from build123d import *

# Parameters (mm, degrees)
SKETCH1_W                      = 80
SKETCH1_H                      = 12.7
BOSS_EXTRUDE1_DEPTH            = 12.7
M4_CLEARANCE_HOLE1_D           = 4.8
M4_CLEARANCE_HOLE1_CSINK_D     = 4.85
M4_CLEARANCE_HOLE1_CSINK_ANGLE = 100
M8_CLEARANCE_HOLE1_D           = 10
M8_CLEARANCE_HOLE1_CSINK_D     = 10.05
M8_CLEARANCE_HOLE1_CSINK_ANGLE = 100
M5_CLEARANCE_HOLE1_D           = 5.8
M5_CLEARANCE_HOLE1_CSINK_D     = 5.85
M5_CLEARANCE_HOLE1_CSINK_ANGLE = 100


with BuildPart() as part:
    # Sketch1 → Boss-Extrude1 (new body)
    with BuildSketch(Plane(origin=(0, 0, 0), x_dir=(1, 0, 0), z_dir=(0, 1, 0))):
        Rectangle(SKETCH1_W, SKETCH1_H)
    extrude(amount=BOSS_EXTRUDE1_DEPTH)

    # M4 Clearance Hole1 (through all)
    with Locations(Plane(origin=(0, 12.7, 0), x_dir=(1, 0, 0), z_dir=(0, 1, 0))):
        with Locations((-35, 0), (-20, 0)):
            CounterSinkHole(M4_CLEARANCE_HOLE1_D / 2, M4_CLEARANCE_HOLE1_CSINK_D / 2, counter_sink_angle=M4_CLEARANCE_HOLE1_CSINK_ANGLE)

    # M8 Clearance Hole1 (through all)
    with Locations(Plane.XY.offset(6.35)):
        with Locations((-3.5, 6.35), (3.5, 6.35)):
            CounterSinkHole(M8_CLEARANCE_HOLE1_D / 2, M8_CLEARANCE_HOLE1_CSINK_D / 2, counter_sink_angle=M8_CLEARANCE_HOLE1_CSINK_ANGLE)

    # M5 Clearance Hole1 (through all)
    with Locations(Plane(origin=(0, 12.7, 0), x_dir=(1, 0, 0), z_dir=(0, 1, 0))):
        with Locations((35, 0), (20, 0)):
            CounterSinkHole(M5_CLEARANCE_HOLE1_D / 2, M5_CLEARANCE_HOLE1_CSINK_D / 2, counter_sink_angle=M5_CLEARANCE_HOLE1_CSINK_ANGLE)


solid = part.part
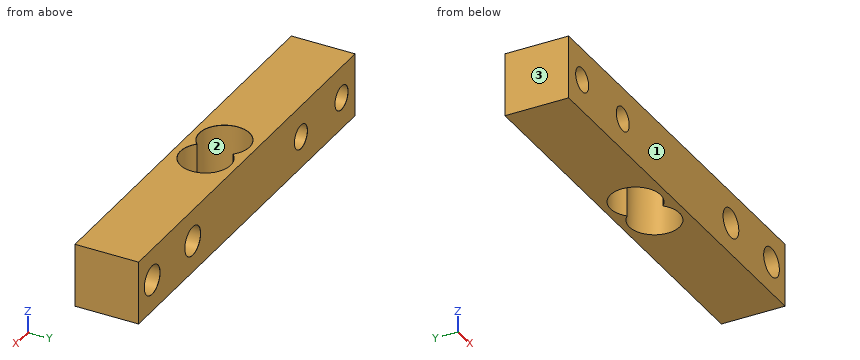
Source: CAD feature listing. Evaluate the final solid. Frame: model axes, mm. Face numbers are marked on the shaded views. Coordinates: 2 decimals unless noted, no trailing zeros. Loops run counter-clockwise (first coordinate to the right, second up) from the corner with the lowest first, then second, coordinate; pieces in that order, holes last. Notation, with made-up numbers: (52.25, 24.25) - (75.25, 24.25) arc R28 cw to (75.25, 57.25) - close; hole circle Ø9 at (60.25, 45). An arc over 180 degrees is marked (long way). One line per question, with ' | ' between items.
1) Section C-C, the plane z = -5. Return loops of the section in (x, y), then the cut area to 3 significant figures.
Report:
outline: (-40, 0) - (40, 0) - (40, 12.7) - (-40, 12.7) - close; hole (0, 2.78) arc R5 ccw (long way) to (0, 9.92) arc R5 ccw (long way) to start | area: 874 mm²
2) Line query: line 1 along X through (y, z) = (5.5, -0.25); line 2 along Y through (x, z) = (-3.5, -1); line 3 along X through (y, z) = (6.35, 3). Output: solid intervals per line, ascending.
Report:
line 1: x = -40 to -37.39, -32.61 to -22.39, -17.61 to -8.43, 8.43 to 17.11, 22.89 to 32.11, 37.89 to 40 | line 2: y = 0 to 1.35, 11.35 to 12.7 | line 3: x = -40 to -8.5, 8.5 to 40
3) Pull-direction query (Y, two-part tool) for the marked faces 1, 2 and 3; classes: released by +Y, released by -Y, zero draft, split by the parting line, or undercut.
Report:
face 1: released by -Y | face 2: undercut | face 3: zero draft
4) Section A-A, the plane y = 6.35. Return loops of the section in (x, z) (3 decimals).
Report:
outline: (-40, -6.35) - (-8.5, -6.35) - (-8.5, 6.329) - (-8.525, 6.35) - (-40, 6.35) - close; (8.5, -6.35) - (40, -6.35) - (40, 6.35) - (8.525, 6.35) - (8.5, 6.329) - close; hole circle Ø4.8 at (-35, 0); hole circle Ø4.8 at (-20, 0); hole circle Ø5.8 at (20, 0); hole circle Ø5.8 at (35, 0)
5) First-contact query: P1, Ø5, axis at x = 35, z = 0, coming from the -Y side. Flat tip, straight axial feed; report the tip coordinate or a pass-through.
Report:
P1: passes through
6) Section D-D, the plane x = 3.5. Return loops of the section in (y, z) (3 decimals).
Report:
outline: (0, -6.35) - (1.35, -6.35) - (1.35, 6.329) - (1.325, 6.35) - (0, 6.35) - close; (11.35, -6.35) - (12.7, -6.35) - (12.7, 6.35) - (11.375, 6.35) - (11.35, 6.329) - close
7) Section B-B, the plane x = -20. Return loops of the section in (y, z) (3 decimals), then the cut area to 3 significant figures.
Report:
outline: (0, -6.35) - (12.7, -6.35) - (12.7, -2.425) - (12.679, -2.4) - (0, -2.4) - close; (0, 2.4) - (12.679, 2.4) - (12.7, 2.425) - (12.7, 6.35) - (0, 6.35) - close | area: 100 mm²
